Can you work these out from the drawing? Everything is in mm from the part's minimum corner. A direction names the side the tool comes from. Give positions to 0.01 mm unless a question says otherwise; leave off trailing zeros. Loops run counter-clockwise (first coordinate to the right, second up) from the corner with the lowest first, then second, coordinate; pieces in that order, holes last. Notation, with made-up numbers: (-6.5, 33) -> (11.5, 33) arc R26 ccw to (11.5, 62) -> close; hole circle Ø3 at (16.25, -1). An arc over 180 degrees is marked (long way). Return JSON: item names as keys, results as strings. Group by question number.
Q1. Suppose I cut it at B-B, the plane y = 103.77. Please give me the cut outline in (x, z).
Q2. Suppose I cut it at C-C, the plane y = 3.75. Please give me the cut outline in (x, z).
Q3. Will these pins go through, and if not, where does the flat tip stop? pin 1 (2 mm diameter, centred on x = 101.21, y = 3.75, fed in from +Z); pin 2 (1 mm diameter, centred on x = 84, z = 25.5, fed in from +Y); pin 3 (4 mm diameter, centred on x = 52.5, z = 48, fed in from -Y); pin 4 (15 mm diameter, centred on y = 6, z = 21.5, fed in from -X).
Q4. Suppose I cut it at D-D, the plane z = 40.5. Please give me the cut outline in (x, y), and give its area (3 significant figures).
Q5. Suppose I cut it at A-A, the plane x = 3.75. Please give me the cut outline in (y, z).
Q6. Which directions (+Z, -Z, +X, -X, +Y, -Y) give clear straight access to the entire face, cutting with the end or side of a thin tool? Please do the marked faces 1, 2 and 3.
Q7. I need wall thicknesses on line 1 along Y through (x, z) = (101.21, 46.45); line 2 along X through (y, z) = (3, 48); line 3 along X through (y, z) = (103, 46). Which ranges of each line are inside material? Lowest first, please. Write a range as [from, to].
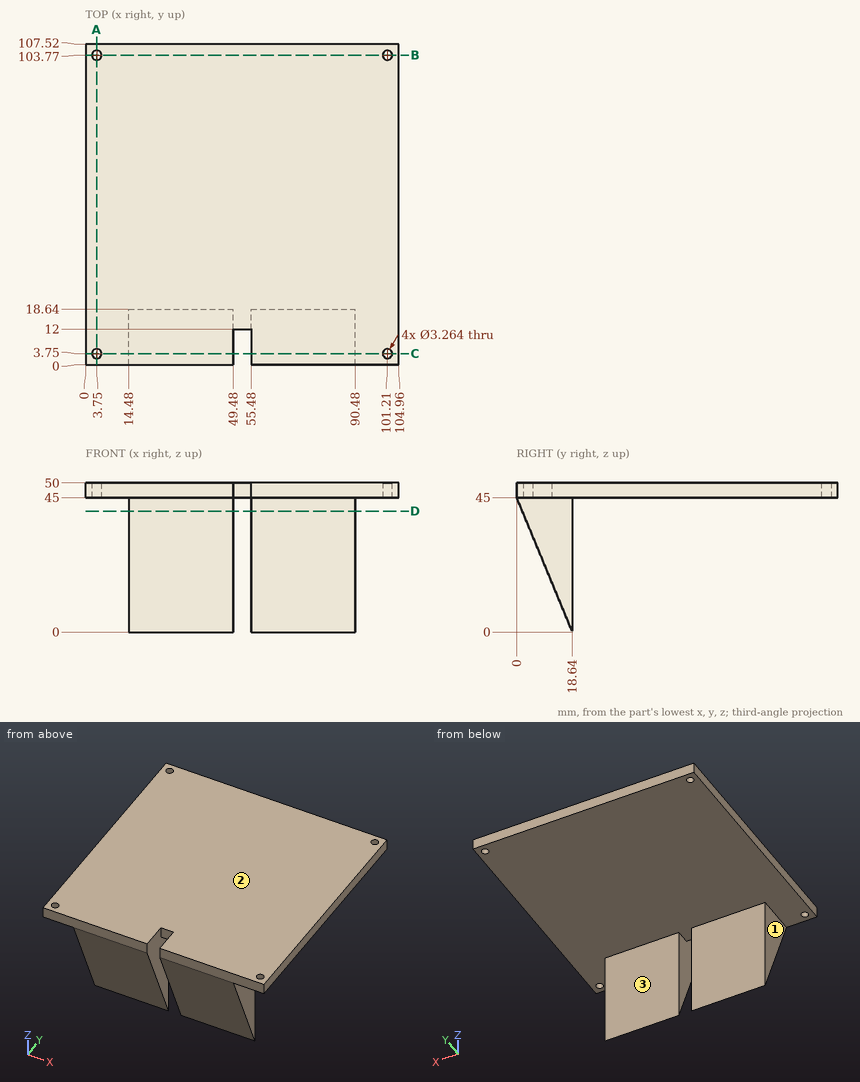
Ans:
{
 "1": {"outline": "(0, 45) -> (2.12, 45) -> (2.12, 50) -> (0, 50) -> close; (5.38, 45) -> (99.58, 45) -> (99.58, 50) -> (5.38, 50) -> close; (102.84, 45) -> (104.96, 45) -> (104.96, 50) -> (102.84, 50) -> close"},
 "2": {"outline": "(0, 45) -> (2.12, 45) -> (2.12, 50) -> (0, 50) -> close; (5.38, 45) -> (14.48, 45) -> (14.48, 35.95) -> (49.48, 35.95) -> (49.48, 50) -> (5.38, 50) -> close; (55.48, 35.95) -> (90.48, 35.95) -> (90.48, 45) -> (99.58, 45) -> (99.58, 50) -> (55.48, 50) -> close; (102.84, 45) -> (104.96, 45) -> (104.96, 50) -> (102.84, 50) -> close"},
 "3": {"pin 1": "passes through", "pin 2": "stops at y = 18.64", "pin 3": "stops at y = 12", "pin 4": "stops at x = 14.48"},
 "4": {"outline": "(14.48, 1.86) -> (49.48, 1.86) -> (49.48, 18.64) -> (14.48, 18.64) -> close; (55.48, 1.86) -> (90.48, 1.86) -> (90.48, 18.64) -> (55.48, 18.64) -> close", "area": "1,170 mm^2"},
 "5": {"outline": "(0, 45) -> (2.12, 45) -> (2.12, 50) -> (0, 50) -> close; (5.38, 45) -> (102.14, 45) -> (102.14, 50) -> (5.38, 50) -> close; (105.4, 45) -> (107.52, 45) -> (107.52, 50) -> (105.4, 50) -> close"},
 "6": {"face 1": "-Z, -X, +Y, -Y", "face 2": "+Z, +X, -X, +Y, -Y", "face 3": "-Z, +X, -X, +Y"},
 "7": {"line 1": "y = [0, 2.12], [5.38, 102.14], [105.4, 107.52]", "line 2": "x = [0, 2.3], [5.2, 49.48], [55.48, 99.76], [102.66, 104.96]", "line 3": "x = [0, 2.31], [5.19, 99.77], [102.65, 104.96]"}
}
